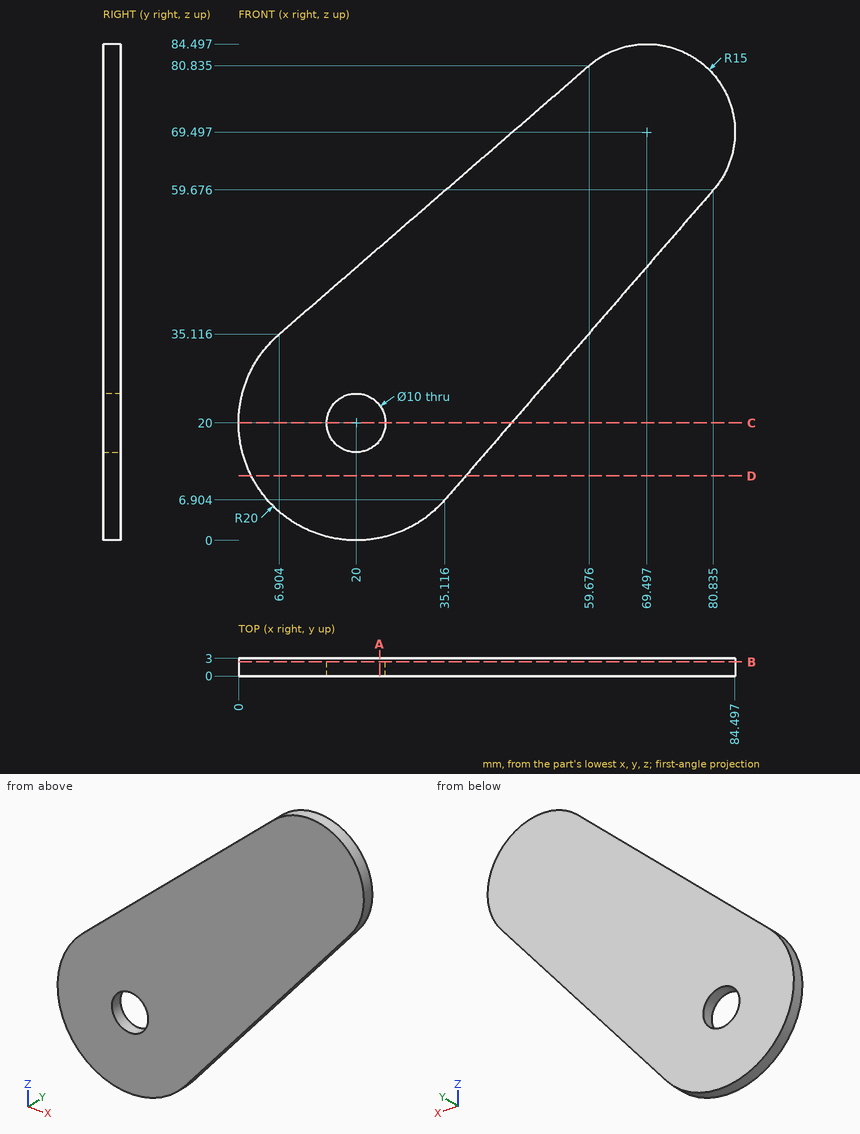
The figure shows three views and two pictorial views of one solid part (mm, origin at its lowest corner). Answer the questions. Round coordinates to 2 decimals unless told otherwise and drop trailing zeros. Write each loop counter-clockwise with the first axis right and the second up, starting at its lowest first coordinate (ties: lowest second). Pieces come first, ordered by that corner, then holes. Notation, with made-up numbers: M 34,0.5 L 87,0.5 A12 cw 87,19.5 Z; hole C 65,-38 d4. An arc over 180 degrees is marked long. Write each question's results on one line, items separated by ' | '. Start each with the question number.
(1) The part is cut by section C-C, the plane z = 20. Write down the section's boundary in (x, y), and give its area (3 significant figures).
(2) Find the intervals of material crossed by line 1 (X direction, y = 2.4, z = 20); line 2 (Z direction, x = 39, y = 2.55) (1 decimal); line 3 (X direction, y = 2.65, z = 15.5) (1 decimal), in increasing order.
(3) Each of these flat-tipped pins is pushed along its axis until it touches: P1, Ø1, axis at x = 41.5, y = 1, coming from the -Z side (1 decimal); P2, Ø13, axis at x = 20, z = 20, coming from the +Y side. Where does it stop, or does it pass through?
(4) The part is cut by section D-D, the plane z = 11. Write down the section's boundary in (x, y) (1 decimal), and give its area (3 significant figures).
(5) The part is cut by section B-B, the plane y = 2.4. Write down the section's boundary in (x, z) (1 decimal).
(6) The part is cut by section A-A, the plane x = 24. Write down the section's boundary in (y, z) (1 decimal).
Worked answers:
1) outline: M 0,0 L 15,0 L 15,3 L 0,3 Z; M 25,0 L 46.46,0 L 46.46,3 L 25,3 Z | area: 109 mm²
2) line 1: x = 0 to 15, 25 to 46.46 | line 2: z = 11.4 to 62.9 | line 3: x = 0.5 to 17.8, 22.2 to 42.6
3) P1: stops at z = 13.7 | P2: stops at y = 3
4) outline: M 2.1,0 L 38.7,0 L 38.7,3 L 2.1,3 Z | area: 110 mm²
5) outline: M 6.9,35.1 A20 ccw long 35.1,6.9 L 80.8,59.7 A15 ccw 59.7,80.8 Z; hole C 20,20 d10
6) outline: M 0,0.4 L 3,0.4 L 3,17 L 0,17 Z; M 0,23 L 3,23 L 3,49.9 L 0,49.9 Z
